from build123d import *

# Parameters (mm, degrees)
BOSS_EXTRUDE1_DEPTH = 31.75
BOSS_EXTRUDE2_DEPTH = 2.54
FILLET1_R           = 5.715
FILLET3_SIZE        = 6.35
FILLET3_SIZE_2      = 2.54
CUT_EXTRUDE1_DEPTH  = 109.038210315


with BuildPart() as part:
    # Sketch1 → Boss-Extrude1 (new body)
    with BuildSketch(Plane(origin=(0, 0, 0), x_dir=(1, 0, 0), z_dir=(0, 1, 0))):
        with BuildLine():
            Line((-52.3875, 23.8125), (52.3875, 23.8125))
            ThreePointArc((52.3875, 23.8125), (56.877628061, 21.952628061), (58.7375, 17.4625))
            Line((58.7375, 17.4625), (58.7375, -17.4625))
            ThreePointArc((58.7375, -17.4625), (56.877628061, -21.952628061), (52.3875, -23.8125))
            Line((52.3875, -23.8125), (-52.3875, -23.8125))
            ThreePointArc((-52.3875, -23.8125), (-56.877628061, -21.952628061), (-58.7375, -17.4625))
            Line((-58.7375, -17.4625), (-58.7375, 17.4625))
            ThreePointArc((-58.7375, 17.4625), (-56.877628061, 21.952628061), (-52.3875, 23.8125))
        make_face()
        with BuildLine():
            Line((-56.1975, 17.4625), (-56.1975, -17.4625))
            ThreePointArc((-56.1975, -17.4625), (-55.081576836, -20.156576836), (-52.3875, -21.2725))
            Line((-52.3875, -21.2725), (52.3875, -21.2725))
            ThreePointArc((52.3875, -21.2725), (55.081576836, -20.156576836), (56.1975, -17.4625))
            Line((56.1975, -17.4625), (56.1975, 17.4625))
            ThreePointArc((56.1975, 17.4625), (55.081576836, 20.156576836), (52.3875, 21.2725))
            Line((52.3875, 21.2725), (-52.3875, 21.2725))
            ThreePointArc((-52.3875, 21.2725), (-55.081576836, 20.156576836), (-56.1975, 17.4625))
        make_face(mode=Mode.SUBTRACT)
    extrude(amount=BOSS_EXTRUDE1_DEPTH)

    # Sketch2 → Boss-Extrude2 (add)
    with BuildSketch(Plane(origin=(0, 31.75, 0), x_dir=(1, 0, 0), z_dir=(0, 1, 0))):
        with BuildLine():
            Line((-65.0875, -42.8625), (65.0875, -42.8625))
            ThreePointArc((65.0875, -42.8625), (74.067756121, -39.142756121), (77.7875, -30.1625))
            Line((77.7875, -30.1625), (77.7875, 30.1625))
            ThreePointArc((77.7875, 30.1625), (74.067756121, 39.142756121), (65.0875, 42.8625))
            Line((65.0875, 42.8625), (-65.0875, 42.8625))
            ThreePointArc((-65.0875, 42.8625), (-74.067756121, 39.142756121), (-77.7875, 30.1625))
            Line((-77.7875, 30.1625), (-77.7875, -30.1625))
            ThreePointArc((-77.7875, -30.1625), (-74.067756121, -39.142756121), (-65.0875, -42.8625))
        make_face()
        with BuildLine():
            Line((52.3875, 21.2725), (-52.3875, 21.2725))
            ThreePointArc((-52.3875, 21.2725), (-55.081576836, 20.156576836), (-56.1975, 17.4625))
            Line((-56.1975, 17.4625), (-56.1975, -17.4625))
            ThreePointArc((-56.1975, -17.4625), (-55.081576836, -20.156576836), (-52.3875, -21.2725))
            Line((-52.3875, -21.2725), (52.3875, -21.2725))
            ThreePointArc((52.3875, -21.2725), (55.081576836, -20.156576836), (56.1975, -17.4625))
            Line((56.1975, -17.4625), (56.1975, 17.4625))
            ThreePointArc((56.1975, 17.4625), (55.081576836, 20.156576836), (52.3875, 21.2725))
        make_face(mode=Mode.SUBTRACT)
    extrude(amount=BOSS_EXTRUDE2_DEPTH)

    # Fillet1
    fillet1_edges = [part.edges().sort_by_distance(p)[0] for p in [
        (-56.877628061, 31.75, -21.952628061),
        (-58.7375, 31.75, 0),
        (-56.877628061, 31.75, 21.952628061),
        (0, 31.75, 23.8125),
        (56.877628061, 31.75, 21.952628061),
        (58.7375, 31.75, 0),
        (56.877628061, 31.75, -21.952628061),
        (0, 31.75, -23.8125),
    ]]
    fillet(fillet1_edges, radius=FILLET1_R)

    # Fillet3
    # an asymmetric fillet: 6.35, 2.54 mm, written as the material it takes off along each edge
    with BuildSketch(Plane(origin=(-52.3875, 34.29, 21.2725), x_dir=(0, -1, 0), z_dir=(1, 0, 0)), Plane(origin=(52.3875, 34.29, -21.2725), x_dir=(0, -1, 0), z_dir=(-1, 0, 0))) as fillet3_piece_1:
        with BuildLine():
            Bezier((FILLET3_SIZE, 0), (0, 0), (0, -FILLET3_SIZE_2), weights=[1, 0.707106781, 1])
            Line((0, -FILLET3_SIZE_2), (0, 0))
            Line((0, 0), (FILLET3_SIZE, 0))
        make_face()
    extrude(amount=104.775, mode=Mode.SUBTRACT)
    with BuildSketch(Plane(origin=(52.3875, 34.29, 17.4625), x_dir=(0, 0, 1), z_dir=(-1, 0, 0))) as fillet3_piece_2:
        with BuildLine():
            Bezier((3.81, -FILLET3_SIZE), (3.81, 0), (3.81 + FILLET3_SIZE_2, 0), weights=[1, 0.707106781, 1])
            Line((3.81 + FILLET3_SIZE_2, 0), (3.81, 0))
            Line((3.81, 0), (3.81, -FILLET3_SIZE))
        make_face()
    revolve(axis=Axis((52.3875, 34.29, 17.4625), (0, 1, 0)), revolution_arc=90, mode=Mode.SUBTRACT)
    with BuildSketch(Plane(origin=(-52.3875, 34.29, 17.4625), x_dir=(-1, 0, 0), z_dir=(0, 0, -1))) as fillet3_piece_3:
        with BuildLine():
            Bezier((3.81, -FILLET3_SIZE), (3.81, 0), (3.81 + FILLET3_SIZE_2, 0), weights=[1, 0.707106781, 1])
            Line((3.81 + FILLET3_SIZE_2, 0), (3.81, 0))
            Line((3.81, 0), (3.81, -FILLET3_SIZE))
        make_face()
    revolve(axis=Axis((-52.3875, 34.29, 17.4625), (0, 1, 0)), revolution_arc=90, mode=Mode.SUBTRACT)
    with BuildSketch(Plane(origin=(56.1975, 34.29, 17.4625), x_dir=(0, -1, 0), z_dir=(0, 0, -1)), Plane(origin=(-56.1975, 34.29, -17.4625), x_dir=(0, -1, 0), z_dir=(0, 0, 1))) as fillet3_piece_4:
        with BuildLine():
            Bezier((FILLET3_SIZE, 0), (0, 0), (0, -FILLET3_SIZE_2), weights=[1, 0.707106781, 1])
            Line((0, -FILLET3_SIZE_2), (0, 0))
            Line((0, 0), (FILLET3_SIZE, 0))
        make_face()
    extrude(amount=34.925, mode=Mode.SUBTRACT)
    with BuildSketch(Plane(origin=(52.3875, 34.29, -17.4625), x_dir=(1, 0, 0), z_dir=(0, 0, 1))) as fillet3_piece_5:
        with BuildLine():
            Bezier((3.81, -FILLET3_SIZE), (3.81, 0), (3.81 + FILLET3_SIZE_2, 0), weights=[1, 0.707106781, 1])
            Line((3.81 + FILLET3_SIZE_2, 0), (3.81, 0))
            Line((3.81, 0), (3.81, -FILLET3_SIZE))
        make_face()
    revolve(axis=Axis((52.3875, 34.29, -17.4625), (0, 1, 0)), revolution_arc=90, mode=Mode.SUBTRACT)
    with BuildSketch(Plane(origin=(-52.3875, 34.29, -17.4625), x_dir=(0, 0, -1), z_dir=(1, 0, 0))) as fillet3_piece_6:
        with BuildLine():
            Bezier((3.81, -FILLET3_SIZE), (3.81, 0), (3.81 + FILLET3_SIZE_2, 0), weights=[1, 0.707106781, 1])
            Line((3.81 + FILLET3_SIZE_2, 0), (3.81, 0))
            Line((3.81, 0), (3.81, -FILLET3_SIZE))
        make_face()
    revolve(axis=Axis((-52.3875, 34.29, -17.4625), (0, 1, 0)), revolution_arc=90, mode=Mode.SUBTRACT)

    # Sketch3 → Cut-Extrude1 (cut, through all)
    with BuildSketch(Plane.XY.offset(23.8125)):
        with BuildLine():
            Line((-52.3875, 0), (-52.3875, 5.03908358))
            ThreePointArc((-52.3875, 5.03908358), (-55.566366011, 5.675815064), (-58.7375, 6.35))
            Line((-58.7375, 6.35), (-58.7375, 0))
            Line((-58.7375, 0), (-52.3875, 0))
        make_face()
        with BuildLine():
            ThreePointArc((-8.980256121, 0), (-8.954247565, 0.07262614), (-8.927651669, 0.145039258))
            ThreePointArc((-8.927651669, 0.145039258), (-30.755078825, 1.726220229), (-52.3875, 5.03908358))
            Line((-52.3875, 5.03908358), (-52.3875, 0))
            Line((-52.3875, 0), (-8.980256121, 0))
        make_face()
        with BuildLine():
            ThreePointArc((-1.188e-06, 0), (4.464414281, 0.036262197), (8.927651669, 0.145039258))
            ThreePointArc((8.927651669, 0.145039258), (0, 6.35), (-8.927651669, 0.145039258))
            ThreePointArc((-8.927651669, 0.145039258), (-4.464415469, 0.036262216), (-1.188e-06, 0))
        make_face()
        with BuildLine():
            ThreePointArc((8.980256121, 0), (8.954247565, 0.07262614), (8.927651669, 0.145039258))
            ThreePointArc((8.927651669, 0.145039258), (4.464414281, 0.036262197), (-1.188e-06, 0))
            Line((-1.188e-06, 0), (8.980256121, 0))
        make_face()
        with BuildLine():
            ThreePointArc((-1.188e-06, 0), (-4.464415469, 0.036262216), (-8.927651669, 0.145039258))
            ThreePointArc((-8.927651669, 0.145039258), (-8.954247565, 0.07262614), (-8.980256121, 0))
            Line((-8.980256121, 0), (-1.188e-06, 0))
        make_face()
        with BuildLine():
            Line((52.3875, 0), (52.3875, 5.03908358))
            ThreePointArc((52.3875, 5.03908358), (30.755078825, 1.726220229), (8.927651669, 0.145039258))
            ThreePointArc((8.927651669, 0.145039258), (8.954247565, 0.07262614), (8.980256121, 0))
            Line((8.980256121, 0), (52.3875, 0))
        make_face()
        with BuildLine():
            Line((58.7375, 0), (58.7375, 6.35))
            ThreePointArc((58.7375, 6.35), (55.566366011, 5.675815064), (52.3875, 5.03908358))
            Line((52.3875, 5.03908358), (52.3875, 0))
            Line((52.3875, 0), (58.7375, 0))
        make_face()
    extrude(amount=-CUT_EXTRUDE1_DEPTH, mode=Mode.SUBTRACT)


solid = part.part
Input: part model. Units: mm. Frame: model coordinates. A direction names the side the tool comes from. Coordinates: 2 decimals unless noted, no trailing zeros. Loops run counter-clockwise (first coordinate to the right, second up) from the corner with the lowest first, then second, coordinate; pieces in that order, holes last. Notation, with made-up numbers: (-29.75, 82.25) -> (-20.75, 82.25) arc R23 ccw to (-20.75, 112.25) -> close; hole circle Ø6 at (54.25, 51). An arc over 180 degrees is marked (long way). One line per item, written item: value.
(1) Set-up query: faces 4 (the face through (56.93, 15.39, 21.9)), 5 (the face through (1, 13, 23.812)), 6 (the face through (56.198, 17, 0)). Return all of +Z, -Z, +X, -X, +Y, -Y with unobstructed straight access to the full face (end or side cutting, diameter ignored); none if empty.
Answer below:
face 4: +Z, +X, -Y
face 5: +Z, +X, -X, -Y
face 6: +Y, -Y
(2) Pin query (flat end, axial travel): pin 1 Ø8 at (y, z) = (13, -17) entering from +X; pin 2 Ø10 at (y, z) = (16.5, -2) entering from -X; pin 3 Ø13 at (x, y) = (12, 16.5) entering from +Z. Return the tip coordinate at first contact, or that it passes through.
Answer below:
pin 1: stops at x = 58.74
pin 2: stops at x = -58.74
pin 3: stops at z = 23.81
(3) Cut plane C-C (z = 36). Output: boundary loops of the cut face in (x, y).
Answer below:
outline: (-76.37, 31.75) -> (76.37, 31.75) -> (76.37, 34.29) -> (-76.37, 34.29) -> close
(4) Draft query along Z for faces 1 (the face through (-1, 14, 21.272)), 2 (the face through (-58.738, 16, 0)), 3 (the face through (73.97, 33, 39.24)). Return one class per face: pulls with the +Z half, pulls with the -Z half, needs draft (parallel to the pull), parting line crosses it, or undercut.
Answer below:
face 1: undercut
face 2: needs draft
face 3: pulls with the +Z half
(5) Ray query, line 1 along Z through (x, y) = (10.5, 8); line 2 along X through (y, z) = (17.5, 17); line 3 along Y through (x, z) = (15, 32.5). Return the intervals inside material, ascending.
Answer below:
line 1: z = -23.81 to -21.27, 21.27 to 23.81
line 2: x = -58.74 to -56.2, 56.2 to 58.74
line 3: y = 31.75 to 34.29
(6) Cut plane A-A (y = 24.5). Output: boundary loops of the cut face in (x, z).
Answer below:
outline: (-58.74, -17.46) arc R6.35 ccw to (-52.39, -23.81) -> (52.39, -23.81) arc R6.35 ccw to (58.74, -17.46) -> (58.74, 17.46) arc R6.35 ccw to (52.39, 23.81) -> (-52.39, 23.81) arc R6.35 ccw to (-58.74, 17.46) -> close; hole (-56.2, -17.46) arc R3.81 ccw to (-52.39, -21.27) -> (52.39, -21.27) arc R3.81 ccw to (56.2, -17.46) -> (56.2, 17.46) arc R3.81 ccw to (52.39, 21.27) -> (-52.39, 21.27) arc R3.81 ccw to (-56.2, 17.46) -> close
